from build123d import *

# Parameters (mm, degrees)
BOSS_EXTRUDE1_DEPTH      = 2
BOSS_EXTRUDE2_DEPTH      = 8
SKETCH24_R               = 3.9
BOSS_EXTRUDE5_DEPTH      = 4.4
SKETCH30_W               = 4.40861202
SKETCH30_H               = 1.324178481
CUT_EXTRUDE12_DEPTH      = 16
CUT_EXTRUDE11_DEPTH      = 23.928148639
FILLET1_R                = 1.5
SKETCH34_R               = 0.75
CUT_EXTRUDE13_DEPTH      = 8
SKETCH35_R               = 0.75
CUT_EXTRUDE14_DEPTH      = 3
CUT_EXTRUDE14_DEPTH_BACK = 8
SKETCH36_R               = 0.95
CUT_EXTRUDE15_DEPTH      = 8
SKETCH37_R               = 2
CUT_EXTRUDE16_DEPTH      = 4.5
SKETCH38_W               = 3
SKETCH38_H               = 1.25
CUT_EXTRUDE17_DEPTH      = 3.6


with BuildPart() as part:
    # Sketch2 → Boss-Extrude1 (new body)
    with BuildSketch(Plane.XY):
        with BuildLine():
            Line((-2.5, 7.5), (-16.7, 7.5))
            Line((-16.7, 7.5), (-20.7, 3.793442666))
            Line((-20.7, 3.793442666), (-20.7, -4.031648778))
            Line((-20.7, -4.031648778), (-15.7, -7.5))
            Line((-15.7, -7.5), (-6.7, -7.5))
            Line((-6.7, -7.5), (-4.2, -5.6))
            ThreePointArc((-4.2, -5.6), (3.130495168, -6.260990337), (7, 0))
            ThreePointArc((7, 0), (4.949747468, 4.949747468), (0, 7))
            Line((0, 7), (0, 7.5))
            Line((0, 7.5), (-2.5, 7.5))
        make_face()
    extrude(amount=BOSS_EXTRUDE1_DEPTH)

    # Sketch4 → Boss-Extrude2 (add)
    with BuildSketch(Plane.XY.offset(2)):
        Polygon((-15.7, -7.5), (-6.7, -7.5), (-6.759079174, -4.5), (-7.7, -4.5), (-7.7, 2), (-5.5, 2), (-5.5, 5.3), (-2.5, 5.3), (-2.5, 7.5), (-16.7, 7.5), (-20.7, 3.793442666), (-20.7, -4.031648778), align=None)
    extrude(amount=BOSS_EXTRUDE2_DEPTH)

    # Sketch24 → Boss-Extrude5 (add)
    with BuildSketch(Plane.XY.offset(2)):
        Circle(SKETCH24_R)
    extrude(amount=BOSS_EXTRUDE5_DEPTH)

    # Sketch30 → Cut-Extrude12 (cut)
    with BuildSketch(Plane(origin=(-5.5, 0, 0), x_dir=(0, 0, -1), z_dir=(1, 0, 0))):
        with Locations((-4.20430601, 4.63791076)):
            Rectangle(SKETCH30_W, SKETCH30_H)
    extrude(amount=-CUT_EXTRUDE12_DEPTH, mode=Mode.SUBTRACT)

    # Sketch28 → Cut-Extrude11 (cut, through all)
    with BuildSketch(Plane.XY.offset(6.4)):
        with BuildLine():
            Line((-1, 1.732050808), (-1, -1.732050808))
            ThreePointArc((-1, -1.732050808), (2, 0), (-1, 1.732050808))
        make_face()
    extrude(amount=-CUT_EXTRUDE11_DEPTH, mode=Mode.SUBTRACT)

    # Fillet1
    # the kernel refuses this fillet: 1.5 mm, written as the material it takes off along each edge
    with BuildSketch(Plane(origin=(-15.230677435, -6, 1.5), x_dir=(-0.5699665637840448, -0.8216678867816415, 0), z_dir=(0, 0, -1))) as fillet1_piece_1_section:
        Polygon((0, 0), (FILLET1_R * 1.02, 0), (FILLET1_R * 1.02, -FILLET1_R * 0.319139344377), (FILLET1_R * 0.838101244517, -FILLET1_R * 0.58136589506), align=None)
    fillet1_piece_1 = extrude(amount=FILLET1_R * 1.02, mode=Mode.PRIVATE)
    fillet1_piece_1 = fillet1_piece_1 - Plane(origin=(-15.230677435, -6, 1.5), x_dir=(0.29860685961507855, 0.9543762064253388, 0), z_dir=(0, 0, -1)) * Sphere(FILLET1_R, mode=Mode.PRIVATE)
    add(fillet1_piece_1, mode=Mode.SUBTRACT)
    with BuildSketch(Plane(origin=(-16.11186344, 6, 1.5), x_dir=(-0.6796897201843015, 0.7334997506991983, 0), z_dir=(0, 0, -1))) as fillet1_piece_2_section:
        Polygon((0, 0), (FILLET1_R * 1.02, 0), (FILLET1_R * 1.02, FILLET1_R * 0.399932860855), (FILLET1_R * 0.748169745713, FILLET1_R * 0.693283514588), align=None)
    fillet1_piece_2 = extrude(amount=FILLET1_R * 1.02, mode=Mode.PRIVATE)
    fillet1_piece_2 = fillet1_piece_2 - Plane(origin=(-16.11186344, 6, 1.5), x_dir=(0.3650344157067945, -0.9309940254102596, 0), z_dir=(0, 0, -1)) * Sphere(FILLET1_R, mode=Mode.PRIVATE)
    add(fillet1_piece_2, mode=Mode.SUBTRACT)
    with BuildSketch(Plane(origin=(-19.2, 3.138411196, 1.5), x_dir=(-0.6796897201843015, 0.7334997506991983, 0), z_dir=(0, 0, -1))) as fillet1_piece_3_section:
        Polygon((0, 0), (FILLET1_R * 1.02, 0), (FILLET1_R * 1.02, -FILLET1_R * 0.445421399395), (FILLET1_R * 0.693283514588, -FILLET1_R * 0.748169745713), align=None)
    fillet1_piece_3 = extrude(amount=FILLET1_R * 1.02, mode=Mode.PRIVATE)
    fillet1_piece_3 = fillet1_piece_3 - Plane(origin=(-19.2, 3.138411196, 1.5), x_dir=(0.9164304993244992, -0.40019387789901173, 0), z_dir=(0, 0, -1)) * Sphere(FILLET1_R, mode=Mode.PRIVATE)
    add(fillet1_piece_3, mode=Mode.SUBTRACT)
    with BuildSketch(Plane(origin=(-19.2, -3.246599046, 1.5), x_dir=(-0.5699665637840448, -0.8216678867816415, 0), z_dir=(0, 0, -1))) as fillet1_piece_4_section:
        Polygon((0, 0), (FILLET1_R * 1.02, 0), (FILLET1_R * 1.02, FILLET1_R * 0.533833817771), (FILLET1_R * 0.58136589506, FILLET1_R * 0.838101244517), align=None)
    fillet1_piece_4 = extrude(amount=FILLET1_R * 1.02, mode=Mode.PRIVATE)
    fillet1_piece_4 = fillet1_piece_4 - Plane(origin=(-19.2, -3.246599046, 1.5), x_dir=(0.8859928227090906, 0.46369895202380795, 0), z_dir=(0, 0, -1)) * Sphere(FILLET1_R, mode=Mode.PRIVATE)
    add(fillet1_piece_4, mode=Mode.SUBTRACT)
    with BuildSketch(Plane(origin=(-15.230677435, -7.5, 0), x_dir=(0, 1, 0), z_dir=(1, 0, 0))) as fillet1_piece_5_section:
        with BuildLine():
            CenterArc((FILLET1_R, FILLET1_R), FILLET1_R, 180, 90)
            Line((0, FILLET1_R), (0, 0))
            Line((0, 0), (FILLET1_R, 0))
        make_face()
    fillet1_piece_5 = extrude(amount=12.280677435, mode=Mode.PRIVATE)
    fillet1_piece_5 = split(fillet1_piece_5, bisect_by=Plane(origin=(-9.092127217, -9.318016685, 0.3282266), z_dir=(-0.6050832675335577, 0.7961621941231027, 0)), keep=Keep.TOP, mode=Mode.PRIVATE)
    add(fillet1_piece_5, mode=Mode.SUBTRACT)
    with BuildSketch(Plane(origin=(3.75, 7.5, 0), x_dir=(0, 0, 1), z_dir=(-1, 0, 0))) as fillet1_piece_6:
        with BuildLine():
            CenterArc((FILLET1_R, -FILLET1_R), FILLET1_R, 90, 90)
            Line((0, -FILLET1_R), (0, 0))
            Line((0, 0), (FILLET1_R, 0))
        make_face()
    extrude(amount=19.86186344, mode=Mode.SUBTRACT)
    with BuildSketch(Plane(origin=(-17.13139802, 7.100249626, 0), x_dir=(0.6796897201843014, -0.7334997506991981, 0), z_dir=(-0.7334997506991983, -0.6796897201843015, 0))) as fillet1_piece_7:
        with BuildLine():
            CenterArc((FILLET1_R, FILLET1_R), FILLET1_R, 180, 90)
            Line((0, FILLET1_R), (0, 0))
            Line((0, 0), (FILLET1_R, 0))
        make_face()
    extrude(amount=4.21013989, mode=Mode.SUBTRACT)
    with BuildSketch(Plane(origin=(-20.054949846, -4.479100876, 0), x_dir=(0.5699665637840448, 0.8216678867816416, 0), z_dir=(0.8216678867816415, -0.5699665637840448, 0))) as fillet1_piece_8:
        with BuildLine():
            CenterArc((FILLET1_R, FILLET1_R), FILLET1_R, 180, 90)
            Line((0, FILLET1_R), (0, 0))
            Line((0, 0), (FILLET1_R, 0))
        make_face()
    extrude(amount=4.830811364, mode=Mode.SUBTRACT)
    with BuildSketch(Plane(origin=(-20.7, 3.138411196, 0), x_dir=(1, 0, 0), z_dir=(0, -1, 0))) as fillet1_piece_9:
        with BuildLine():
            CenterArc((FILLET1_R, FILLET1_R), FILLET1_R, 180, 90)
            Line((0, FILLET1_R), (0, 0))
            Line((0, 0), (FILLET1_R, 0))
        make_face()
    extrude(amount=6.385010242, mode=Mode.SUBTRACT)
    with BuildSketch(Plane(origin=(-15.7, -7.5, 1.5), x_dir=(1, 0, 0), z_dir=(0, 0, 1))) as fillet1_piece_10:
        with BuildLine():
            CenterArc((FILLET1_R * 0.312881710173, FILLET1_R), FILLET1_R, 235.252105822, 34.747894178)
            Line((-FILLET1_R * 0.257084853611, FILLET1_R * 0.178332113218), (0, 0))
            Line((0, 0), (FILLET1_R * 0.312881710173, 0))
        make_face()
    extrude(amount=9.673306413, mode=Mode.SUBTRACT)
    with BuildSketch(Plane(origin=(-20.7, -4.031648778, 1.5), x_dir=(0, 1, 0), z_dir=(0, 0, 1))) as fillet1_piece_11:
        with BuildLine():
            CenterArc((FILLET1_R * 0.523366488011, -FILLET1_R), FILLET1_R, 90, 55.252105822)
            Line((-FILLET1_R * 0.298301398771, -FILLET1_R * 0.430033436216), (0, 0))
            Line((0, 0), (FILLET1_R * 0.523366488011, 0))
        make_face()
    extrude(amount=10.46262433, mode=Mode.SUBTRACT)
    with BuildSketch(Plane(origin=(-20.7, 3.793442666, 1.5), x_dir=(0.7334997506991984, 0.6796897201843014, 0), z_dir=(0, 0, 1))) as fillet1_piece_12:
        with BuildLine():
            CenterArc((FILLET1_R * 0.436687646465, -FILLET1_R), FILLET1_R, 90, 47.18059856)
            Line((-FILLET1_R * 0.296812104234, -FILLET1_R * 0.320310279816), (0, 0))
            Line((0, 0), (FILLET1_R * 0.436687646465, 0))
        make_face()
    extrude(amount=10.137578674, mode=Mode.SUBTRACT)
    with BuildSketch(Plane(origin=(-16.7, 7.5, 1.5), x_dir=(1, 0, 0), z_dir=(0, 0, 1))) as fillet1_piece_13:
        with BuildLine():
            CenterArc((FILLET1_R * 0.392091040054, -FILLET1_R), FILLET1_R, 90, 42.81940144)
            Line((-FILLET1_R * 0.287598680131, -FILLET1_R * 0.266500249301), (0, 0))
            Line((0, 0), (FILLET1_R * 0.392091040054, 0))
        make_face()
    extrude(amount=9.9703414, mode=Mode.SUBTRACT)

    # Sketch34 → Cut-Extrude13 (cut, along a direction that is not the sketch's normal)
    with BuildSketch(Plane.XZ.offset(-2)):
        with Locations((-7, 10)):
            Circle(SKETCH34_R)
    extrude(amount=-CUT_EXTRUDE13_DEPTH, dir=(0.6685833876565112, -0.7436371788377336, 0), mode=Mode.SUBTRACT)

    # Sketch35 → Cut-Extrude14 (cut, two sides, along a direction that is not the sketch's normal)
    with BuildSketch(Plane(origin=(0, -4.5, 0), x_dir=(1, 0, 0), z_dir=(0, 1, 0))) as cut_extrude14_sk:
        with Locations((-8.259079174, -10)):
            Circle(SKETCH35_R)
    extrude(amount=CUT_EXTRUDE14_DEPTH, dir=(0.5999194182208608, 0.8000604299935998, 0), mode=Mode.SUBTRACT)
    extrude(cut_extrude14_sk.sketch, amount=-CUT_EXTRUDE14_DEPTH_BACK, dir=(0.5999194182208608, 0.8000604299935998, 0), mode=Mode.SUBTRACT)

    # Sketch36 → Cut-Extrude15 (cut)
    with BuildSketch(Plane.XY.offset(10)):
        with Locations((-11.7, 0)):
            Circle(SKETCH36_R)
        with Locations((-16.7, 0)):
            Circle(SKETCH36_R)
    extrude(amount=-CUT_EXTRUDE15_DEPTH, mode=Mode.SUBTRACT)

    # Sketch37 → Cut-Extrude16 (cut)
    with BuildSketch(Plane(origin=(0, 0, 0), x_dir=(-1, 0, 0), z_dir=(0, 0, -1))):
        with Locations((11.7, 0)):
            Circle(SKETCH37_R)
        with Locations((16.7, 0)):
            Circle(SKETCH37_R)
    extrude(amount=-CUT_EXTRUDE16_DEPTH, mode=Mode.SUBTRACT)

    # Sketch38 → Cut-Extrude17 (cut)
    with BuildSketch(Plane.XY.offset(10)):
        with Locations((-4, 5.925)):
            Rectangle(SKETCH38_W, SKETCH38_H)
    extrude(amount=-CUT_EXTRUDE17_DEPTH, mode=Mode.SUBTRACT)


with BuildPart() as body_2:
    # Split1: the piece on the far side of the plane
    add(part.part)
    split(bisect_by=Plane.XY.offset(6.4), keep=Keep.BOTTOM)


with BuildPart() as part_1:
    add(part.part)

    # Split1
    split(bisect_by=Plane.XY.offset(6.4), keep=Keep.TOP)


solid = body_2.part
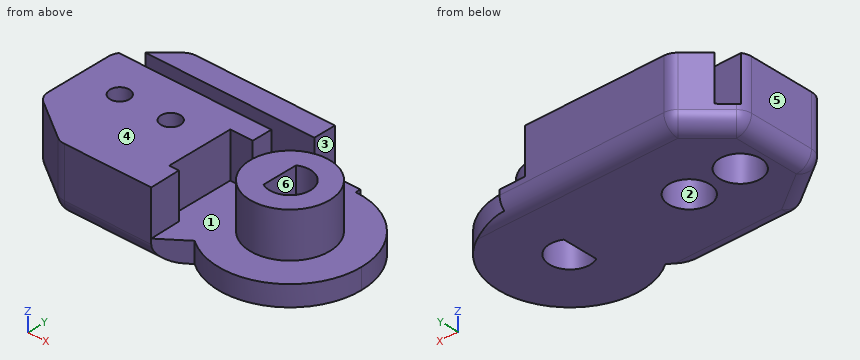
Could you check a few things on this model? Use its own coordinates, in mm. Face numbers are marked on the shaded views. A direction names the side the tool comes from. Give positions to 0.01 mm unless a question says otherwise; leave off trailing zeros. Order: outer loops, then holes, each group sorted by start corner. A loop starts at its lowest first (then second) coordinate and runs counter-clockwise, first axis right, second up.
1. Thinking about a two-plate mould opening in X: for the marked faces 4, 5 and 6, which applies, +X half, -X half, draft (parallel to the pull), parting line (faces both ways), or undercut?
Answers below:
face 4: draft
face 5: -X half
face 6: undercut
2. Which directions (+Z, -Z, +X, -X, +Y, -Y) give clear straight access to the entire face, cutting with the end or side of a thin tool? Please do the marked faces 1, 2 and 3.
Answers below:
face 1: +Z
face 2: -Z
face 3: +Z, +X, +Y
3. I need wall thicknesses on L1, parallel to X at y = 1.5, z = 3; L2, parallel to X at y = -0.5, z = 3.25; L3, parallel to Y at x = 0, z = 2.25. Which ranges of each line are inside material? Lowest first, please.
Answers below:
L1: x = -20.7 to -18.02, -15.38 to -13.02, -10.38 to -7.7, -3.6 to -1, 1.32 to 3.6
L2: x = -20.7 to -18.64, -14.76 to -13.64, -9.76 to -7.7, -3.87 to -1, 1.94 to 3.87
L3: y = -3.9 to -2, 2 to 3.9
4. Suppose I cut it at D-D (z = 1). Write out the boundary of the cut face in (x, y).
Answers below:
outline: (-20.61, -3.25) arc R1.41 ccw to (-20.01, -4.41) - (-16.04, -7.16) arc R1.41 ccw to (-15.23, -7.41) - (-6.59, -7.41) - (-4.2, -5.6) arc R7 ccw (long way) to (0, 7) - (0, 7.41) - (-16.11, 7.41) arc R1.41 ccw to (-17.07, 7.04) - (-20.16, 4.18) arc R1.41 ccw to (-20.61, 3.14) - close; hole circle Ø4 at (-16.7, 0); hole circle Ø4 at (-11.7, 0); hole (-1, -1.73) arc R2 ccw (long way) to (-1, 1.73) - close
5. Suppose I cut it at C-C (x = -12). Write out the boundary of the cut face in (y, z), plus the area to 3 significant figures.
Answers below:
outline: (-7.5, 1.5) arc R1.5 ccw to (-6, 0) - (-1.98, 0) - (-1.98, 4.5) - (-0.9, 4.5) - (-0.9, 6.4) - (-7.5, 6.4) - close; (0.9, 4.5) - (1.98, 4.5) - (1.98, 0) - (6, 0) arc R1.5 ccw to (7.5, 1.5) - (7.5, 6.4) - (5.3, 6.4) - (5.3, 2) - (3.98, 2) - (3.98, 6.4) - (0.9, 6.4) - close
area: 68.0 mm2
6. Suppose I cut it at A-A (z = 3.5). Write out the boundary of the cut face in (x, y), plus the area to 3 significant figures.
Answers below:
outline: (-20.7, -3.25) arc R1.5 ccw to (-20.05, -4.48) - (-16.09, -7.23) arc R1.5 ccw to (-15.23, -7.5) - (-6.7, -7.5) - (-6.76, -4.5) - (-7.7, -4.5) - (-7.7, 2) - (-5.5, 2) - (-5.5, 3.98) - (-20.44, 3.98) arc R1.5 ccw to (-20.7, 3.14) - close; (-19.07, 5.3) - (-2.5, 5.3) - (-2.5, 7.5) - (-16.11, 7.5) arc R1.5 ccw to (-17.13, 7.1) - close; circle Ø7.8 at (0, 0); hole circle Ø4 at (-16.7, 0); hole circle Ø4 at (-11.7, 0); hole (-1, -1.73) arc R2 ccw (long way) to (-1, 1.73) - close
area: 194 mm2
7. For pin 1 (1.5 mm diameter, centred on y = 5.5, z = 1.5, fed in from +X); pin 2 (3 mm diameter, centred on y = 0, z = 3, fed in from +X); pin 3 (2 mm diameter, centred on y = 3, z = 3.5, fed in from +X); pin 4 (1 mm diameter, centred on x = -6, y = -3, fed in from +Z), each with a flat end and sliding along its axis, tell me the tip position at first contact or that it passes through.
Answers below:
pin 1: stops at x = 5.14
pin 2: stops at x = 7
pin 3: stops at x = 3.35
pin 4: stops at z = 2
8. Suppose I cut it at B-B (x = -8). Write out the boundary of the cut face in (y, z).
Answers below:
outline: (-7.5, 1.5) arc R1.5 ccw to (-6, 0) - (6, 0) arc R1.5 ccw to (7.5, 1.5) - (7.5, 6.4) - (5.3, 6.4) - (5.3, 2) - (3.98, 2) - (3.98, 6.4) - (-7.5, 6.4) - close
